```python
from build123d import *

# Parameters (mm, degrees)
SKETCH1_W           = 10
SKETCH1_H           = 5
BOSS_EXTRUDE1_DEPTH = 10.5
SKETCH2_W           = 2.2
SKETCH2_H           = 2.5
BOSS_EXTRUDE2_DEPTH = 0.5
CHAMFER1_SIZE       = 0.5
SKETCH4_R           = 0.25
BOSS_EXTRUDE3_DEPTH = 2.2


with BuildPart() as part:
    # Sketch1 → Boss-Extrude1 (new body)
    with BuildSketch(Plane.XY):
        Rectangle(SKETCH1_W, SKETCH1_H)
    extrude(amount=-BOSS_EXTRUDE1_DEPTH)

    # Sketch2 → Boss-Extrude2 (add)
    with BuildSketch(Plane.XY):
        with Locations((-3.9, 0)):
            Rectangle(SKETCH2_W, SKETCH2_H)
        with Locations((3.9, 0)):
            Rectangle(SKETCH2_W, SKETCH2_H)
    extrude(amount=BOSS_EXTRUDE2_DEPTH)

    # Chamfer1
    chamfer1_edges = [part.edges().sort_by_distance(p)[0] for p in [
        (2.8, 0, 0),
        (-2.8, 0, 0),
    ]]
    chamfer(chamfer1_edges, length=CHAMFER1_SIZE - 0.0001)  # a hair under: the kernel refuses the full size

    # Sketch4 → Boss-Extrude3 (add)
    with BuildSketch(Plane.XY.offset(0.5)):
        with Locations((-3.75, 0.065947188)):
            Circle(SKETCH4_R)
        with Locations(Location((3.75, 0.065947188, 0), (0, 0, 180))):
            Circle(SKETCH4_R)
    extrude(amount=BOSS_EXTRUDE3_DEPTH)


solid = part.part
```
Part model, mm, in its own coordinate system. A direction names the side the tool comes from. Round coordinates to 2 decimals unless told otherwise and drop trailing zeros. Loops run counter-clockwise (first coordinate to the right, second up) from the corner with the lowest first, then second, coordinate; pieces in that order, holes last. Notation, with made-up numbers: (-14.75, -30) -> (36.25, -30) arc R21 ccw to (36.25, -18) -> close; hole circle Ø3 at (82.5, 27). An arc over 180 degrees is marked (long way). Use one line per item in the form item = value. Start each with the question number.
Item 1: Band-saw the part on D-D (x = 2.5). List the corners of the cut face in (y, z).
Item 2: Band-saw the part on A-A (x = 3.75). List the corners of the cut face in (y, z).
Item 3: Tool access for faces 1 (the flat face through (-5, 0, -5)), 2 (the flat face through (0, 0, 0)): list every direction of +Z, -Z, +X, -X, +Y, -Y with a clear straight run to the whole face (end or side of a thin tool).
Item 4: Band-saw the part on C-C (z = 1.75). List the corners of the cut face in (x, y).
Item 5: Drop a flat-ended pin along its axis: pin 1 Ø0.7 at (x, y) = (-4.5, 0) entering from +Z. Give the stop position or say it passes through.
Item 6: Drill centre lines: line 1 along Z through (x, y) = (1.5, 0.25); line 2 along Z through (x, y) = (4.25, -0.8). Where is each one in solid material? Low to high.
Data:
q1.outline = (-2.5, -10.5) -> (2.5, -10.5) -> (2.5, 0) -> (1.25, 0) -> (1.25, 0.2) -> (-1.25, 0.2) -> (-1.25, 0) -> (-2.5, 0) -> close
q2.outline = (-2.5, -10.5) -> (2.5, -10.5) -> (2.5, 0) -> (1.25, 0) -> (1.25, 0.5) -> (0.32, 0.5) -> (0.32, 2.7) -> (-0.18, 2.7) -> (-0.18, 0.5) -> (-1.25, 0.5) -> (-1.25, 0) -> (-2.5, 0) -> close
q3.face_1 = +Z, -Z, -X, +Y, -Y
q3.face_2 = +Z
q4.outline = circle Ø0.5 at (-3.75, 0.07); circle Ø0.5 at (3.75, 0.07)
q5.pin_1 = 0.5
q6.line_1 = -10.5 to 0
q6.line_2 = -10.5 to 0.5
